Source: CAD feature listing. Evaluate the final solid. Frame: model axes, mm. Give positions to 0.01 mm unless a question says otherwise; leave off trailing zeros. Order: outer loops, then holes, each group sorted by start corner. A loop starts at its lowest first (then second) coordinate and runs counter-clockwise, first axis right, second up.
```python
from build123d import *

# Parameters (mm, degrees)
F0_R     = 13.69544
F1_DEPTH = 25.4


with BuildPart() as f1:
    # F0 (on Top) → F1 (new body)
    with BuildSketch(Plane.XY):
        Polygon((0, 55.732161), (-39.546929, 19.697119), (37.409257, 20.307882), align=None)
        Polygon((-39.546929, 19.697119), (-39.546929, -47.486853), (37.409257, -47.486853), (37.409257, 20.307882), align=None)
        with Locations((0, -26.415514)):
            Circle(F0_R, mode=Mode.SUBTRACT)
    extrude(amount=F1_DEPTH)


solid = f1.part
```
1) Material intervals for L1, parallel to Y at x = 0, z = 13.5; L2, parallel to Y at x = 7.5, z = 2.25; L3, parallel to X at y = -39, z = 20.25, sorted ascending.
Report:
L1: y = -47.49 to -40.11, -12.72 to 55.73
L2: y = -47.49 to -37.87, -14.96 to 48.63
L3: x = -39.55 to -5.4, 5.4 to 37.41
2) Draft query along Y for faces 1 (the flat face through (-19.497, 37.967, 12.522)), 2 (the flat face through (-2, -47.487, 13)), 3 (the flat face through (37.409, -14, 13)), 4 (the cylindrical face through (-1.783, -12.837, 12.522)). Return one class per face: +Y half, -Y half, draft (parallel to the pull), parting line (faces both ways), or undercut.
Report:
face 1: +Y half
face 2: -Y half
face 3: draft
face 4: undercut
3) Section query A-A, the plane y = -37.5. Return the cut outline in (x, z).
Report:
outline: (-39.55, 0) - (-8.04, 0) - (-8.04, 25.4) - (-39.55, 25.4) - close; (8.04, 0) - (37.41, 0) - (37.41, 25.4) - (8.04, 25.4) - close
4) Section query C-C, the plane z = 18.75. Return the cut outline in (x, y).
Report:
outline: (-39.55, -47.49) - (37.41, -47.49) - (37.41, 20.31) - (0, 55.73) - (-39.55, 19.7) - close; hole circle Ø27.39 at (0, -26.42)
5) Pin query (flat end, axial travel): pin 1 (12 mm diameter, centred on x = 6.5, z = 8, fed in from +Y); pin 2 (1 mm diameter, centred on x = 16.5, z = 8.5, fed in from +Y); pin 3 (5 mm diameter, centred on x = 5.5, z = 4.5, fed in from +Y). Return the tip coordinate at first contact, or that it passes through.
Report:
pin 1: stops at y = 55.26
pin 2: stops at y = 40.58
pin 3: stops at y = 52.89
6) Section query B-B, the plane x = -6. Return the cut outline in (y, z).
Report:
outline: (-47.49, 0) - (-38.73, 0) - (-38.73, 25.4) - (-47.49, 25.4) - close; (-14.1, 0) - (50.26, 0) - (50.26, 25.4) - (-14.1, 25.4) - close
7) Section query D-D, the plane x = -28.5. Return the cut outline in (y, z).
Report:
outline: (-47.49, 0) - (29.76, 0) - (29.76, 25.4) - (-47.49, 25.4) - close
